Geometry check sheet. Reference: the model listing, model coordinates, mm. Face numbers are marked on the shaded views. A direction names the side the tool comes from. Round coordinates to 2 decimals unless told otherwise and drop trailing zeros. Write each loop counter-clockwise with the first axis right and the second up, starting at its lowest first coordinate (ties: lowest second). Pieces come first, ordered by that corner, then holes.
Item 1: Cross-section at B-B (z = 5). Enter the section's corners in (x, y), then the cut area to 3 significant figures.
Item 2: Cross-section at D-D (z = 18.5). Enter the section's corners in (x, y), then the cut area to 3 significant figures.
Item 3: Draft check along Y on the marked faces 1, 2 and 3. Enter one of: pulls with the +Y half, pulls with the -Y half, needs draft (parallel to the pull), parting line crosses it, or undercut.
Item 4: Cross-section at A-A (x = 1.5). Enter the section's corners in (y, z).
Item 5: Access from +Z, -Z, +X, -X, +Y, -Y to the whole of each face (thin tool, end or side, straight path). Record for the marked faces 4 and 5.
Item 6: Scan lines: probe 1 along Z at (x, y) = (-24, -22); probe 2 along X at (y, z) = (-14.5, 5); probe 3 along Y at (x, z) = (36, 31.5). Record each from-to range of solid material in increasing order.
Item 7: Cross-section at C-C (y = 23.5). Enter the section's corners in (x, z).
Item 8: Depth check by flat-ended pin: P1, Ø1.5, axis at x = -3.5, z = 22.5, coming from the -Y side. Enter the tip coordinate at first touch or a pass-through.
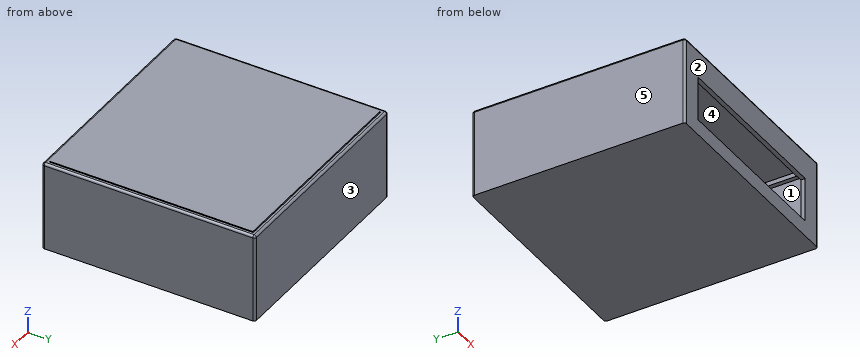
from build123d import *

# Parameters (mm, degrees)
F0_W      = 99
F0_H      = 96
F0_W_2    = 95
F0_H_2    = 92
F1_DEPTH  = 40
F2_DEPTH  = 2
F3_W      = 80
F3_H      = 20
F4_DEPTH  = 2
F5_R      = 1
F6_W      = 94
F6_H      = 2
F7_DEPTH  = 4
F8_W      = 94
F8_H      = 2
F9_DEPTH  = 4
F10_W     = 94.5
F10_H     = 91.5
F11_DEPTH = 4


with BuildPart() as f1:
    # F0 (on Top) → F1 (new body)
    with BuildSketch(Plane.XY):
        Rectangle(F0_W, F0_H)
        Rectangle(F0_W_2, F0_H_2, mode=Mode.SUBTRACT)
    extrude(amount=F1_DEPTH)

    # F0 (on Top) → F2 (join)
    with BuildSketch(Plane.XY):
        Rectangle(F0_W_2, F0_H_2)
    extrude(amount=F2_DEPTH)

    # F3 (on face) → F4 (cut)
    with BuildSketch(Plane.XZ.offset(48)):
        with Locations((0, 17)):
            Rectangle(F3_W, F3_H)
    extrude(amount=-F4_DEPTH, mode=Mode.SUBTRACT)

    # F5
    f5_edges = [f1.edges().sort_by_distance(p)[0] for p in [
        (-49.5, 0, 40),
        (0, -48, 40),
        (49.5, 0, 40),
        (0, 48, 40),
        (-49.5, -48, 20),
        (49.5, -48, 20),
        (49.5, 48, 20),
        (-49.5, 48, 20),
    ]]
    fillet(f5_edges, radius=F5_R)

    # F6 (on face) → F7 (join)
    with BuildSketch(Plane(origin=(-49.5, 0, 0), x_dir=(0, -1, 0), z_dir=(-1, 0, 0))):
        with Locations((0, 35)):
            Rectangle(F6_W, F6_H)
    extrude(amount=-F7_DEPTH)

    # F8 (on face) → F9 (join)
    with BuildSketch(Plane.YZ.offset(49.5)):
        with Locations((0, 35)):
            Rectangle(F8_W, F8_H)
    extrude(amount=-F9_DEPTH)

    # F10 (on face) → F11 (join)
    with BuildSketch(Plane.XY.offset(36)):
        with Locations((-0.25, -0.25)):
            Rectangle(F10_W, F10_H)
    extrude(amount=F11_DEPTH)


solid = f1.part
Resolved:
1. outline: (-49.5, -47) arc R1 ccw to (-48.5, -48) - (48.5, -48) arc R1 ccw to (49.5, -47) - (49.5, 47) arc R1 ccw to (48.5, 48) - (-48.5, 48) arc R1 ccw to (-49.5, 47) - close; hole (-47.5, -46) - (47.5, -46) - (47.5, 46) - (-47.5, 46) - close
1. area: 763 mm2
2. outline: (-49.5, -47) arc R1 ccw to (-48.5, -48) - (-40, -48) - (-40, -46) - (-47.5, -46) - (-47.5, 46) - (47.5, 46) - (47.5, -46) - (40, -46) - (40, -48) - (48.5, -48) arc R1 ccw to (49.5, -47) - (49.5, 47) arc R1 ccw to (48.5, 48) - (-48.5, 48) arc R1 ccw to (-49.5, 47) - close
2. area: 603 mm2
3. face 1: undercut
3. face 2: pulls with the -Y half
3. face 3: pulls with the +Y half
4. outline: (-48, 0) - (48, 0) - (48, 39) arc R1 ccw to (47, 40) - (46, 40) - (46, 2) - (-46, 2) - (-46, 7) - (-48, 7) - close; (-48, 27) - (-46, 27) - (-46, 36) - (45.5, 36) - (45.5, 40) - (-47, 40) arc R1 ccw to (-48, 39) - close
5. face 4: none
5. face 5: +Z, -Z, -X, +Y, -Y
6. probe 1: z = 0 to 2, 36 to 40
6. probe 2: x = -49.5 to -47.5, 47.5 to 49.5
6. probe 3: y = -48 to -46, 46 to 48
7. outline: (-49.5, 0) - (49.5, 0) - (49.5, 39) arc R1 ccw to (48.5, 40) - (47.5, 40) - (47.5, 36) - (47, 36) - (47, 40) - (-48.5, 40) arc R1 ccw to (-49.5, 39) - close; hole (-47.5, 2) - (47.5, 2) - (47.5, 34) - (45.5, 34) - (45.5, 36) - (-45.5, 36) - (-45.5, 34) - (-47.5, 34) - close
8. P1: stops at y = 46
